Verification items for the finished model (mm, model axes). Coordinates: 2 decimals unless noted, no trailing zeros. Write each loop counter-clockwise with the first axis right and the second up, starting at its lowest first coordinate (ties: lowest second). Pieces come first, ordered by that corner, then holes. Notation, with made-up numbers: M 58.5,32 L 77.5,32 A34 cw 77.5,68 Z; hole C 13,29 d7. An arc over 180 degrees is marked long. Answer in a Markdown table with one row per item.
from build123d import *

# Parameters (mm, degrees)
SKETCH_1_W      = 20
SKETCH_1_H      = 600
EXTRUDE_1_DEPTH = 12


with BuildPart() as part:
    # Эскиз1 → Выдавливание1 (new body)
    with BuildSketch(Plane(origin=(0, 0, 0), x_dir=(-1, 0, 0), z_dir=(0, 1, 0))):
        Polygon((-915, -300), (-915, -610), (915, -610), (915, -300), (895, -300), (895, -590), (-895, -590), (-895, -300), align=None)
        Polygon((-895, 300), (-895, 590), (895, 590), (895, 300), (915, 300), (915, 610), (-915, 610), (-915, 300), align=None)
        with Locations((-905, 0)):
            Rectangle(SKETCH_1_W, SKETCH_1_H)
        with Locations((905, 0)):
            Rectangle(SKETCH_1_W, SKETCH_1_H)
    extrude(amount=EXTRUDE_1_DEPTH)


solid = part.part
1) Sectioned sample at A-A (x = -742). Record the cut outline in (y, z).
Response values:
| item | result |
|---|---|
| outline | M 0,-610 L 12,-610 L 12,-590 L 0,-590 Z; M 0,590 L 12,590 L 12,610 L 0,610 Z |
2) Sectioned sample at C-C (z = -368). Record the cut outline in (x, y).
Response values:
| item | result |
|---|---|
| outline | M -915,0 L -895,0 L -895,12 L -915,12 Z; M 895,0 L 915,0 L 915,12 L 895,12 Z |
3) Thickness scan on L1, parallel to X at y = 5.25, z = 21; L2, parallel to Z at x = 535.5, y = 10.5. Record the ranges inside material, lowest first. Write a range as [from, to].
Response values:
| item | result |
|---|---|
| L1 | x = [-915, -895], [895, 915] |
| L2 | z = [-610, -590], [590, 610] |
4) Sectioned sample at B-B (y = 8). Record the cut outline in (x, z), then the cut area to 3 significant figures.
Response values:
| item | result |
|---|---|
| outline | M -915,-610 L 915,-610 L 915,610 L -915,610 Z; hole M -895,-590 L 895,-590 L 895,590 L -895,590 Z |
| area | 120,000 mm² |
